Work out the finished part from the listing and answer in its coordinate system (mm). A direction names the side the tool comes from. Coordinates: 2 decimals unless noted, no trailing zeros. Order: outer loops, then holes, each group sorted by start corner. A loop starts at its lowest first (then second) coordinate and runs counter-clockwise, first axis right, second up.
1. Determine the mould class of faces 4 (the flat face through (25, 8.755, -40)), 5 (the cylindrical face through (12.627, -7.14, -13.032)), 6 (the flat face through (12, 2.755, 2)), 7 (the cylindrical face through (7.571, 7.825, -5.992)) for opening direction Y: +Y half, -Y half, draft (parallel to the pull), parting line (faces both ways), or undercut.
2. The part is cut by section B-B, the plane x = 7.5. Count the separate pieces of the cut face and the enclosed holes in it, then the cut area to 3 significant figures.
3. Find the intervals of material crossed by probe 1 along X at (y, z) = (0, 4.5); probe 2 along Z at (x, y) = (22, 10); probe 3 along Z at (x, y) = (22.5, -9), in increasing order.
4. The part is cut by section D-D, the plane z = -12. Give the vertices of the cut face in (x, y) (3 decimals).
5. The part is cut by section C-C, the plane y = -14. Give the vertices of the cut face in (x, z).
6. Flat-ended cylindrical pins translate along their axes: pin 1 Ø3 at (x, z) = (21.5, -40) entering from +Y; pin 2 Ø5 at (x, z) = (13.5, -41) entering from -Y; pin 3 Ø6 at (x, y) = (15, -7.24) entering from -Z. Find the tip coordinate at first contact, or state that the pin passes through.
7. The part is cut by section A-A, the plane z = 5. Give the vertices of the cut face in (x, y) (3 decimals).
8. A tool of negligible diameter and unlimited length cuts with its end or side. For faces 1 (the flat face through (1, -7, 2)), 2 (the cylindrical face through (22.429, 7.825, 10.506)), 3 (the flat face through (5, -7, -32.243)), from which of +Z, -Z, +X, -X, +Y, -Y can it reach the whole face along a straight path? Write none if from no direction.
```python
from build123d import *
from OCP.BRepFilletAPI import BRepFilletAPI_MakeChamfer

# Parameters (mm, degrees)
RESSALTO_EXTRUS_O1_DEPTH = 30
CORTE_EXTRUS_O1_REACH    = 68.527
ESBO_O2_R                = 2.375
ESBO_O2_3_R              = 4.75
ESBO_O2_3_R_2            = 2.375
CORTE_EXTRUS_O3_DEPTH    = 4
CORTE_EXTRUS_O2_REACH    = 80.086
ESBO_O3_R                = 2.375
ESBO_O3_3_R              = 2.375
CORTE_EXTRUS_O4_DEPTH    = 4
ESBO_O4_W                = 6
ESBO_O4_H                = 6
ESBO_O4_W_2              = 3
RESSALTO_EXTRUS_O2_DEPTH = 1
CORTE_EXTRUS_O5_START    = -10
CORTE_EXTRUS_O5_DEPTH    = 57.527149202
CHANFRO1_SIZE            = 1
ESBO_O6_W                = 10
ESBO_O6_H                = 6
RESSALTO_EXTRUS_O3_DEPTH = 1
CHANFRO2_SIZE            = 0.5
CHANFRO2_SIZE_2          = 1


with BuildPart() as part:
    # Esboço1 → Ressalto-extrusão1 (new body)
    with BuildSketch(Plane(origin=(0, 0, 0), x_dir=(0, 0, -1), z_dir=(1, 0, 0))):
        Polygon((51.243161309, 12.755336939), (-18.756838691, 12.755336939), (-18.756838691, -9.981327227), (-11.493502857, -17.244663061), (31.243161309, -17.244663061), (31.243161309, 2.755336939), (51.243161309, 2.755336939), align=None)
    extrude(amount=RESSALTO_EXTRUS_O1_DEPTH)

    # Esboço2 → Corte-extrusão1 (cut, up to next)
    with BuildSketch(Plane(origin=(0, 12.755336939, 0), x_dir=(1, 0, 0), z_dir=(0, 1, 0)), mode=Mode.PRIVATE) as corte_extrus_o1_sk1:
        with Locations(Location((7.5, 41.243161309, 0), (0, 0, 270))):
            Circle(ESBO_O2_R)
    corte_extrus_o1_tool1 = extrude(corte_extrus_o1_sk1.sketch, amount=-CORTE_EXTRUS_O1_REACH, mode=Mode.PRIVATE) & part.part
    # Esboço2 → Corte-extrusão1 (cut, up to next)
    with BuildSketch(Plane(origin=(0, 12.755336939, 0), x_dir=(1, 0, 0), z_dir=(0, 1, 0)), mode=Mode.PRIVATE) as corte_extrus_o1_sk2:
        with Locations(Location((22.5, 41.243161309, 0), (0, 0, 270))):
            Circle(ESBO_O2_R)
    corte_extrus_o1_tool2 = extrude(corte_extrus_o1_sk2.sketch, amount=-CORTE_EXTRUS_O1_REACH, mode=Mode.PRIVATE) & part.part
    # Esboço2 → Corte-extrusão1 (cut, up to next)
    with BuildSketch(Plane(origin=(0, 12.755336939, 0), x_dir=(1, 0, 0), z_dir=(0, 1, 0)), mode=Mode.PRIVATE) as corte_extrus_o1_sk3:
        with BuildLine():
            Line((4.25, 2.743161309), (4.25, -7.256838691))
            ThreePointArc((4.25, -7.256838691), (7.5, -10.506838691), (10.75, -7.256838691))
            Line((10.75, -7.256838691), (10.75, 2.743161309))
            ThreePointArc((10.75, 2.743161309), (7.5, 5.993161309), (4.25, 2.743161309))
        make_face()
    corte_extrus_o1_tool3 = extrude(corte_extrus_o1_sk3.sketch, amount=-CORTE_EXTRUS_O1_REACH, mode=Mode.PRIVATE) & part.part
    # Esboço2 → Corte-extrusão1 (cut, up to next)
    with BuildSketch(Plane(origin=(0, 12.755336939, 0), x_dir=(1, 0, 0), z_dir=(0, 1, 0)), mode=Mode.PRIVATE) as corte_extrus_o1_sk4:
        with BuildLine():
            Line((19.25, 2.743161309), (19.25, -7.256838691))
            ThreePointArc((19.25, -7.256838691), (22.5, -10.506838691), (25.75, -7.256838691))
            Line((25.75, -7.256838691), (25.75, 2.743161309))
            ThreePointArc((25.75, 2.743161309), (22.5, 5.993161309), (19.25, 2.743161309))
        make_face()
    corte_extrus_o1_tool4 = extrude(corte_extrus_o1_sk4.sketch, amount=-CORTE_EXTRUS_O1_REACH, mode=Mode.PRIVATE) & part.part
    add(corte_extrus_o1_tool1.solids().sort_by_distance((7.5, 12.755337, -41.243161))[0], mode=Mode.SUBTRACT)
    add(corte_extrus_o1_tool2.solids().sort_by_distance((22.5, 12.755337, -41.243161))[0], mode=Mode.SUBTRACT)
    add(corte_extrus_o1_tool3.solids().sort_by_distance((7.5, 12.755337, 2.256839))[0], mode=Mode.SUBTRACT)
    add(corte_extrus_o1_tool4.solids().sort_by_distance((22.5, 12.755337, 2.256839))[0], mode=Mode.SUBTRACT)

    # Esboço2<3> → Corte-extrusão3 (cut)
    # profile 1 of 2: a face of its own
    with BuildSketch(Plane(origin=(0, 12.755336939, 0), x_dir=(1, 0, 0), z_dir=(0, 1, 0))):
        with Locations(Location((7.5, 41.243161309, 0), (0, 0, 270))):
            Circle(ESBO_O2_3_R)
        with Locations(Location((7.5, 41.243161309, 0), (0, 0, 270))):
            Circle(ESBO_O2_3_R_2, mode=Mode.SUBTRACT)
    # profile 2 of 2: a face of its own
    with BuildSketch(Plane(origin=(0, 12.755336939, 0), x_dir=(1, 0, 0), z_dir=(0, 1, 0))):
        with Locations(Location((22.5, 41.243161309, 0), (0, 0, 270))):
            Circle(ESBO_O2_3_R)
        with Locations(Location((22.5, 41.243161309, 0), (0, 0, 270))):
            Circle(ESBO_O2_3_R_2, mode=Mode.SUBTRACT)
    extrude(amount=-CORTE_EXTRUS_O3_DEPTH, mode=Mode.SUBTRACT)

    # Esboço3 → Corte-extrusão2 (cut, up to next)
    with BuildSketch(Plane.XY.offset(18.756838691), mode=Mode.PRIVATE) as corte_extrus_o2_sk1:
        with Locations((15, -7.244663061)):
            Circle(ESBO_O3_R)
    corte_extrus_o2_tool1 = extrude(corte_extrus_o2_sk1.sketch, amount=-CORTE_EXTRUS_O2_REACH, mode=Mode.PRIVATE) & part.part
    add(corte_extrus_o2_tool1.solids().sort_by_distance((15, -7.244663, 18.756839))[0], mode=Mode.SUBTRACT)

    # Esboço3<3> → Corte-extrusão4 (cut)
    # profile 1 of 2: a face of its own
    with BuildSketch(Plane.XY.offset(18.756838691)):
        with BuildLine():
            Line((18.882417963, -9.981327227), (11.117582037, -9.981327227))
            ThreePointArc((11.117582037, -9.981327227), (15, -11.994663061), (18.882417963, -9.981327227))
        make_face()
    # profile 2 of 2: a face of its own
    with BuildSketch(Plane.XY.offset(18.756838691)):
        with BuildLine():
            ThreePointArc((18.882417963, -9.981327227), (19.527912617, -8.680109799), (19.75, -7.244663061))
            ThreePointArc((19.75, -7.244663061), (13.564553262, -2.716750444), (11.117582037, -9.981327227))
            Line((11.117582037, -9.981327227), (18.882417963, -9.981327227))
        make_face()
        with Locations((15, -7.244663061)):
            Circle(ESBO_O3_3_R, mode=Mode.SUBTRACT)
    extrude(amount=-CORTE_EXTRUS_O4_DEPTH, mode=Mode.SUBTRACT)

    # Esboço4 → Ressalto-extrusão2 (add)
    with BuildSketch(Plane.XZ.offset(-2.755336939)):
        with Locations((15, -41.243161309)):
            Rectangle(ESBO_O4_W, ESBO_O4_H)
        with Locations((1.5, -41.243161309)):
            Rectangle(ESBO_O4_W_2, ESBO_O4_H)
        with Locations((28.5, -41.243161309)):
            Rectangle(ESBO_O4_W_2, ESBO_O4_H)
    extrude(amount=RESSALTO_EXTRUS_O2_DEPTH)

    # Esboço2<4> → Corte-extrusão5 (cut, through all)
    # profile 1 of 2: a face of its own
    with BuildSketch(Plane(origin=(0, 12.755336939, 0), x_dir=(1, 0, 0), z_dir=(0, 1, 0)).offset(CORTE_EXTRUS_O5_START)):
        with BuildLine():
            Line((1, 2.743161309), (1, -7.256838691))
            ThreePointArc((1, -7.256838691), (7.5, -13.756838691), (14, -7.256838691))
            Line((14, -7.256838691), (14, 2.743161309))
            ThreePointArc((14, 2.743161309), (7.5, 9.243161309), (1, 2.743161309))
        make_face()
        with BuildLine():
            ThreePointArc((10.75, 2.743161309), (7.5, 5.993161309), (4.25, 2.743161309))
            Line((4.25, 2.743161309), (4.25, -7.256838691))
            ThreePointArc((4.25, -7.256838691), (7.5, -10.506838691), (10.75, -7.256838691))
            Line((10.75, -7.256838691), (10.75, 2.743161309))
        make_face(mode=Mode.SUBTRACT)
    # profile 2 of 2: a face of its own
    with BuildSketch(Plane(origin=(0, 12.755336939, 0), x_dir=(1, 0, 0), z_dir=(0, 1, 0)).offset(CORTE_EXTRUS_O5_START)):
        with BuildLine():
            Line((16, 2.743161309), (16, -7.256838691))
            ThreePointArc((16, -7.256838691), (22.5, -13.756838691), (29, -7.256838691))
            Line((29, -7.256838691), (29, 2.743161309))
            ThreePointArc((29, 2.743161309), (22.5, 9.243161309), (16, 2.743161309))
        make_face()
        with BuildLine():
            ThreePointArc((25.75, 2.743161309), (22.5, 5.993161309), (19.25, 2.743161309))
            Line((19.25, 2.743161309), (19.25, -7.256838691))
            ThreePointArc((19.25, -7.256838691), (22.5, -10.506838691), (25.75, -7.256838691))
            Line((25.75, -7.256838691), (25.75, 2.743161309))
        make_face(mode=Mode.SUBTRACT)
    extrude(amount=-CORTE_EXTRUS_O5_DEPTH, mode=Mode.SUBTRACT)

    # Chanfro1
    chanfro1_edges = [part.edges().sort_by_distance(p)[0] for p in [
        (0, 12.755336939, -16.243161309),
        (30, 12.755336939, -16.243161309),
        (15, 12.755336939, 18.756838691),
        (15, 12.755336939, -51.243161309),
    ]]
    chamfer(chanfro1_edges, length=CHANFRO1_SIZE)

    # Esboço6 → Ressalto-extrusão3 (add)
    with BuildSketch(Plane(origin=(0, 0, -31.243161309), x_dir=(-1, 0, 0), z_dir=(0, 0, -1))):
        with Locations((-25, -7.244663061)):
            Rectangle(ESBO_O6_W, ESBO_O6_H)
        with Locations((-5, -7.244663061)):
            Rectangle(ESBO_O6_W, ESBO_O6_H)
    extrude(amount=RESSALTO_EXTRUS_O3_DEPTH)

    # Chanfro2
    chanfro2_edges_1 = [part.edges().sort_by_distance(p)[0] for p in [
        (25, -4.244663061, -31.243161309),
    ]]
    chanfro2_side_1 = [part.faces().sort_by_distance(p)[0] for p in [
        (25, -4.234663061, -31.243161309),
    ]]
    chanfro2_edges_2 = [part.edges().sort_by_distance(p)[0] for p in [
        (5, -4.244663061, -31.243161309),
    ]]
    chanfro2_side_2 = [part.faces().sort_by_distance(p)[0] for p in [
        (5, -4.234663061, -31.243161309),
    ]]
    chanfro2 = BRepFilletAPI_MakeChamfer(part.part.solid().wrapped)
    for e in chanfro2_edges_1:
        chanfro2.Add(CHANFRO2_SIZE - 0.0001, CHANFRO2_SIZE_2 - 0.0001, e.wrapped, chanfro2_side_1[0].wrapped)
    for e in chanfro2_edges_2:
        chanfro2.Add(CHANFRO2_SIZE - 0.0001, CHANFRO2_SIZE_2 - 0.0001, e.wrapped, chanfro2_side_2[0].wrapped)
    add(Compound.cast(chanfro2.Shape()), mode=Mode.REPLACE)  # a hair under: the kernel refuses the full size


solid = part.part
```
Geometry says:
1. face 4: +Y half
1. face 5: undercut
1. face 6: -Y half
1. face 7: draft
2. separate pieces: 3
2. enclosed holes: 0
2. area: 990 mm2
3. probe 1: x = 0 to 1, 14 to 16, 29 to 30
3. probe 2: z = -51.24 to -45.97, -36.52 to -5.95, 10.47 to 18.76
3. probe 3: z = -32.24 to -9.24, 13.76 to 18.76
4. outline: (0, -17.245) - (30, -17.245) - (30, 11.755) - (29, 12.755) - (1, 12.755) - (0, 11.755) - close; hole circle Ø4.75 at (15, -7.245)
5. outline: (0, -31.24) - (30, -31.24) - (30, 14.74) - (0, 14.74) - close; hole (1, -2.74) arc R6.5 ccw to (14, -2.74) - (14, 7.26) arc R6.5 ccw to (1, 7.26) - close; hole (16, -2.74) arc R6.5 ccw to (29, -2.74) - (29, 7.26) arc R6.5 ccw to (16, 7.26) - close
6. pin 1: stops at y = 8.76
6. pin 2: stops at y = 1.76
6. pin 3: stops at z = -31.24
7. outline: (0, -17.245) - (1, -17.245) - (1, 2.755) - (4.25, 2.755) - (4.25, 12.755) - (1, 12.755) - (0, 11.755) - close; (10.75, 2.755) - (14, 2.755) - (14, -5.09) arc R2.375 cw to (16, -5.09) - (16, 2.755) - (19.25, 2.755) - (19.25, 12.755) - (10.75, 12.755) - close; (14, -17.245) - (16, -17.245) - (16, -9.399) arc R2.375 cw to (14, -9.399) - close; (25.75, 2.755) - (29, 2.755) - (29, -17.245) - (30, -17.245) - (30, 11.755) - (29, 12.755) - (25.75, 12.755) - close
8. face 1: -Y
8. face 2: +Y, -Y
8. face 3: -Z, +X, -X, -Y
